from build123d import *

# Parameters (mm, degrees)
F0_R      = 19.75
F1_DEPTH  = 17
F2_R      = 18.25
F3_DEPTH  = 15
F4_R      = 9.5
F5_DEPTH  = 14.5
F6_R      = 9.25
F7_DEPTH  = 14
F8_R      = 3.25
F9_DEPTH  = 9.5
F10_R     = 1.6
F11_DEPTH = 7
F12_R     = 1.551351
F13_DEPTH = 25.4
F14_DEPTH = 25.4
F15_R     = 2.896187
F16_DEPTH = 1
F17_R     = 1.546412
F18_DEPTH = 1
F19_R     = 0.295483
F20_DEPTH = 0.2


with BuildPart() as f1:
    # F0 (on Front) → F1 (new body)
    with BuildSketch(Plane.XZ):
        Circle(F0_R)
    extrude(amount=F1_DEPTH)

    # F2 (on face) → F3 (cut)
    with BuildSketch(Plane.XZ.offset(17)):
        Circle(F2_R)
    extrude(amount=-F3_DEPTH, mode=Mode.SUBTRACT)

    # F4 (on face) → F5 (join)
    with BuildSketch(Plane(origin=(0, 0, 0), x_dir=(-1, 0, 0), z_dir=(0, 1, 0))):
        Circle(F4_R)
    extrude(amount=-F5_DEPTH)

    # F6 (on face) → F7 (cut)
    with BuildSketch(Plane(origin=(0, 0, 0), x_dir=(-1, 0, 0), z_dir=(0, 1, 0))):
        Circle(F6_R)
    extrude(amount=-F7_DEPTH, mode=Mode.SUBTRACT)

    # F8 (on face) → F9 (join)
    with BuildSketch(Plane.XZ.offset(14.5)):
        Circle(F8_R)
    extrude(amount=F9_DEPTH)

    # F10 (on face) → F11 (cut)
    with BuildSketch(Plane.XZ.offset(24)):
        Circle(F10_R)
    extrude(amount=-F11_DEPTH, mode=Mode.SUBTRACT)

    # F12 (on face) → F13 (cut)
    with BuildSketch(Plane(origin=(0, -14, 0), x_dir=(-1, 0, 0), z_dir=(0, 1, 0))):
        with Locations((0, 4.813187)):
            Circle(F12_R)
    extrude(amount=-F13_DEPTH, mode=Mode.SUBTRACT)

    # F12 (on face) → F14 (cut)
    with BuildSketch(Plane(origin=(0, -14, 0), x_dir=(-1, 0, 0), z_dir=(0, 1, 0))):
        with Locations((-3.403437, 3.403437)):
            Circle(F12_R)
        with Locations((-4.813187, 0)):
            Circle(F12_R)
        with Locations((-3.403437, -3.403437)):
            Circle(F12_R)
        with Locations((0, -4.813187)):
            Circle(F12_R)
        with Locations((3.403437, -3.403437)):
            Circle(F12_R)
        with Locations((4.813187, 0)):
            Circle(F12_R)
        with Locations((3.403437, 3.403437)):
            Circle(F12_R)
    extrude(amount=-F14_DEPTH, mode=Mode.SUBTRACT)

    # F15 (on face) → F16 (join)
    with BuildSketch(Plane(origin=(0, -14, 0), x_dir=(-1, 0, 0), z_dir=(0, 1, 0))):
        Circle(F15_R)
    extrude(amount=F16_DEPTH)

    # F17 (on face) → F18 (join)
    with BuildSketch(Plane(origin=(0, -13, 0), x_dir=(-1, 0, 0), z_dir=(0, 1, 0))):
        Circle(F17_R)
    extrude(amount=F18_DEPTH)

    # F19 (on face) → F20 (join)
    with BuildSketch(Plane(origin=(0, -13, 0), x_dir=(-1, 0, 0), z_dir=(0, 1, 0))):
        with Locations((-1.352597, 1.86169)):
            Circle(F19_R)
        with Locations((0, 2.301175)):
            Circle(F19_R)
        with Locations((1.352597, 1.86169)):
            Circle(F19_R)
        with Locations((2.188547, 0.711102)):
            Circle(F19_R)
        with Locations((2.188547, -0.711102)):
            Circle(F19_R)
        with Locations((1.352597, -1.86169)):
            Circle(F19_R)
        with Locations((0, -2.301175)):
            Circle(F19_R)
        with Locations((-1.352597, -1.86169)):
            Circle(F19_R)
        with Locations((-2.188547, -0.711102)):
            Circle(F19_R)
        with Locations((-2.188547, 0.711102)):
            Circle(F19_R)
    extrude(amount=F20_DEPTH)


solid = f1.part
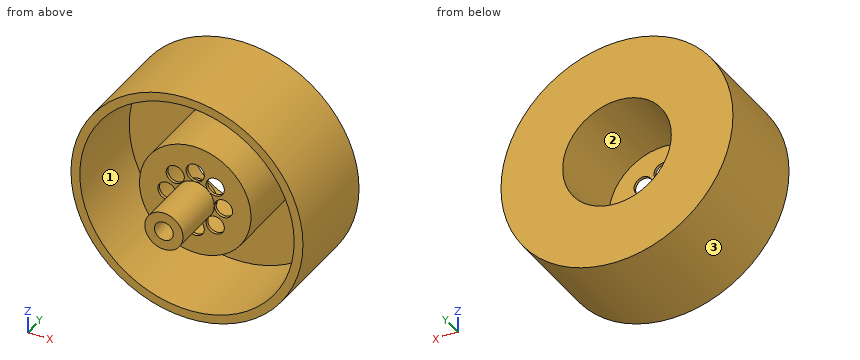
Model file for the job. Use its own axes, mm. Face numbers are marked on the shaded views. A direction names the side the tool comes from. Coordinates: 2 decimals unless noted, no trailing zeros. Order: outer loops, then holes, each group sorted by start corner. A loop starts at its lowest first (then second) coordinate and runs counter-clockwise, first axis right, second up. Notation, with made-up numbers: M -38,44.5 L -31,44.5 A26 cw -31,82.5 Z; hole C 34,1 d10. An arc over 180 degrees is marked long. Return JSON: item names as keys, results as strings.
1. Drill centre lines: probe 1 along Z at (x, y) = (0, -14.2); probe 2 along Z at (x, y) = (0, -21.5); probe 3 along Z at (x, y) = (3, -3.75). Where is each one in solid material? Low to high.
Ans:
{"probe 1": "-19.75 to -18.25, -9.5 to -6.36, -3.26 to 3.26, 6.36 to 9.5, 18.25 to 19.75", "probe 2": "-3.25 to -1.6, 1.6 to 3.25", "probe 3": "-19.52 to -18, -9.01 to -8.75, 8.75 to 9.01, 18 to 19.52"}
2. Saw through at A-A (y = -8.25). Give the cut face in (x, z), and give its area (3 significant figures).
Ans:
{"outline": "C 0,0 d39.5; C 0,0 d19; hole C 0,0 d36.5; hole C 0,0 d18.5", "area": "194 mm^2"}
3. Flat gauge pins, fed straight in: pin 1 (0.5 mm diameter, centred on x = -1.5, z = 2, fed in from +Y); pin 2 (6 mm diameter, centred on x = 4.5, z = -7, fed in from -Y); pin 3 (2 mm diameter, centred on x = 10.5, y = -3, fed in from -Z). Where does each tip first touch, or does it go through?
Ans:
{"pin 1": "y = -12.8", "pin 2": "y = -14.5", "pin 3": "z = -17.32"}
4. Tool access for the marked faces 1, 2 and 3: list every direction of +Z, -Z, +X, -X, +Y, -Y with a clear straight run to the whole face (end or side of a thin tool).
Ans:
{"face 1": "-Y", "face 2": "+Y", "face 3": "+Y, -Y"}
5. Saw through at B-B (z = -5.5). Give the cut face in (x, y), and give its area (3 significant figures).
Ans:
{"outline": "M -18.97,-17 L -17.4,-17 L -17.4,-2 L -7.75,-2 L -7.75,-14.5 L -1.39,-14.5 L -1.39,-14 L -7.44,-14 L -7.44,0 L -18.97,0 Z; M 1.39,-14.5 L 7.75,-14.5 L 7.75,-2 L 17.4,-2 L 17.4,-17 L 18.97,-17 L 18.97,0 L 7.44,0 L 7.44,-14 L 1.39,-14 Z", "area": "107 mm^2"}
6. Saw through at C-C (x = 7.5). Give the cut face in (y, z), and give its area (3 significant figures).
Ans:
{"outline": "M -17,-18.27 L 0,-18.27 L 0,-5.41 L -14,-5.41 L -14,5.41 L 0,5.41 L 0,18.27 L -17,18.27 L -17,16.64 L -2,16.64 L -2,5.83 L -14.5,5.83 L -14.5,-5.83 L -2,-5.83 L -2,-16.64 L -17,-16.64 Z", "area": "116 mm^2"}
7. Saw through at D-D (y = -21.5). Give the cut face in (x, z).
Ans:
{"outline": "C 0,0 d6.5; hole C 0,0 d3.2"}
